Can you work these out from the model? Positions are in its coordinate system, mm. A direction names the side the tool comes from. Coordinates: 2 decimals unless noted, no trailing zeros. Loops run counter-clockwise (first coordinate to the right, second up) from the corner with the lowest first, then second, coordinate; pieces in that order, holes last.
```python
from build123d import *

# Parameters (mm, degrees)
SKETCH_1_W          = 53.5
SKETCH_1_H          = 45
SKETCH_1_R          = 10.25
SKETCH_1_R_2        = 2
SKETCH_1_R_3        = 1.5
EXTRUDE_1_DEPTH     = 5
SKETCH_3_W          = 5
SKETCH_3_H          = 10
EXTRUDE_2_DEPTH     = 5
SKETCH_4_R          = 1.5
SKETCH_4_W          = 10.4
SKETCH_4_H          = 15.4
CUT_EXTRUDE_2_DEPTH = 40.234073202
FILLET_1_R          = 3
FILLET_2_R          = 3


with BuildPart() as part:
    # ｽｹｯﾁ1 → ﾎﾞｽ - 押し出し1 (new body)
    with BuildSketch(Plane(origin=(0, 0, 0), x_dir=(0, 0, -1), z_dir=(1, 0, 0))):
        Rectangle(SKETCH_1_W, SKETCH_1_H)
        with Locations((-6.75, 0)):
            Circle(SKETCH_1_R, mode=Mode.SUBTRACT)
        with Locations((21.75, 17.5)):
            Circle(SKETCH_1_R_2, mode=Mode.SUBTRACT)
        with Locations(Location((21.75, -17.5, 0), (0, 0, 180))):
            Circle(SKETCH_1_R_2, mode=Mode.SUBTRACT)
        with Locations((6.25, 0)):
            Circle(SKETCH_1_R_3, mode=Mode.SUBTRACT)
        with Locations(Location((-19.75, 0, 0), (0, 0, 180))):
            Circle(SKETCH_1_R_3, mode=Mode.SUBTRACT)
        with Locations((-6.75, 13)):
            Circle(SKETCH_1_R_3, mode=Mode.SUBTRACT)
        with Locations(Location((-6.75, -13, 0), (0, 0, 180))):
            Circle(SKETCH_1_R_3, mode=Mode.SUBTRACT)
    extrude(amount=EXTRUDE_1_DEPTH)

    # ｽｹｯﾁ3 → ﾎﾞｽ - 押し出し2 (add)
    with BuildSketch(Plane(origin=(5, 0, 0), x_dir=(0, 0, -1), z_dir=(1, 0, 0))):
        with Locations((-29.25, 17.5)):
            Rectangle(SKETCH_3_W, SKETCH_3_H)
    extrude(amount=-EXTRUDE_2_DEPTH)

    # ｽｹｯﾁ4 → ｶｯﾄ - 押し出し2 (cut, through all)
    with BuildSketch(Plane(origin=(5, 0, 0), x_dir=(0, 0, -1), z_dir=(1, 0, 0))):
        with Locations((-26.75, 17.5)):
            Circle(SKETCH_4_R)
        with Locations((21.75, -5)):
            Rectangle(SKETCH_4_W, SKETCH_4_H)
    extrude(amount=-CUT_EXTRUDE_2_DEPTH, mode=Mode.SUBTRACT)

    # ﾌｨﾚｯﾄ1
    fillet_1_edges = [part.edges().sort_by_distance(p)[0] for p in [
        (2.5, 22.5, 31.75),
        (2.5, 12.5, 31.75),
        (2.5, -22.5, -26.75),
        (2.5, -22.5, 26.75),
        (2.5, 22.5, -26.75),
    ]]
    fillet(fillet_1_edges, radius=FILLET_1_R)

    # ﾌｨﾚｯﾄ2
    fillet_2_edges = [part.edges().sort_by_distance(p)[0] for p in [
        (2.5, 12.5, 26.75),
    ]]
    fillet(fillet_2_edges, radius=FILLET_2_R)


solid = part.part
```
(1) I want a section at D-D on z = -21.75. Write out the boundary of the cut face in (x, y).
Check values:
outline: (0, -22.5) - (5, -22.5) - (5, -19.5) - (0, -19.5) - close; (0, -15.5) - (5, -15.5) - (5, -12.7) - (0, -12.7) - close; (0, 2.7) - (5, 2.7) - (5, 15.5) - (0, 15.5) - close; (0, 19.5) - (5, 19.5) - (5, 22.5) - (0, 22.5) - close
(2) If I drill on probe 1 along Y at (x, z) = (3.9, 19.75); probe 2 along Y at (x, z) = (4.75, -24); probe 3 along Z at (x, y) = (1.4, 18), over which ranges is the centre line in solid material (lowest first)?
Check values:
probe 1: y = -22.5 to -1.5, 1.5 to 22.5
probe 2: y = -22.49 to -12.7, 2.7 to 22.49
probe 3: z = -26.75 to -23.69, -19.81 to 25.34, 28.16 to 31.75
(3) I want a section at B-B on y = -17.5. Write out the boundary of the cut face in (x, z).
Check values:
outline: (0, -26.75) - (5, -26.75) - (5, -23.75) - (0, -23.75) - close; (0, -19.75) - (5, -19.75) - (5, 26.75) - (0, 26.75) - close
(4) I'm going to push flat-ended pins straight in: pin 1 (1.5 mm diameter, centred on x = 2.5, y = -4, fed in from +Z); pin 2 (5 mm diameter, centred on y = -5, z = 25.5, fed in from -X); pin 3 (16.5 mm diameter, centred on y = 0, z = 6.75, fed in from +X); pin 4 (3 mm diameter, centred on x = 2.5, y = -5, fed in from -Z). Where does each tip first touch, or does it pass through?
Check values:
pin 1: stops at z = 26.75
pin 2: stops at x = 0
pin 3: passes through
pin 4: stops at z = -16.55
(5) Which directions (+Z, -Z, +X, -X, +Y, -Y) give clear straight access to the entire face, cutting with the end or side of a thin tool? Please do faces 5 (the flat face through (3, 17, 31.75)), 6 (the flat face through (2, -5, 26.75)).
Check values:
face 5: +Z, +X, -X, +Y, -Y
face 6: +Z, +X, -X, -Y
(6) I want a section at A-A on z = 19.75. Write out the boundary of the cut face in (x, y).
Check values:
outline: (0, -22.5) - (5, -22.5) - (5, -1.5) - (0, -1.5) - close; (0, 1.5) - (5, 1.5) - (5, 22.5) - (0, 22.5) - close
(7) If we mould it in two halves opening along Y, with no side actions, what happens to faces 1 (the flat face through (3, 2.7, -22)), 2 (the flat face through (3, 22.5, 3)), 3 (the cylindrical face through (2.54, -21.6, 25.89)), 4 (the flat face through (2, 11, -26.75))? For each: released by +Y, released by -Y, zero draft, split by the parting line, or undercut.
Check values:
face 1: undercut
face 2: released by +Y
face 3: released by -Y
face 4: zero draft
(8) I want a section at C-C on y = 0. Write out the boundary of the cut face in (x, z).
Check values:
outline: (0, -16.55) - (5, -16.55) - (5, -7.75) - (0, -7.75) - close; (0, -4.75) - (5, -4.75) - (5, -3.5) - (0, -3.5) - close; (0, 17) - (5, 17) - (5, 18.25) - (0, 18.25) - close; (0, 21.25) - (5, 21.25) - (5, 26.75) - (0, 26.75) - close
